Verification items for the finished model (mm, model axes). A direction names the side the tool comes from. Round coordinates to 2 decimals unless told otherwise and drop trailing zeros. Order: outer loops, then holes, each group sorted by start corner. A loop starts at its lowest first (then second) coordinate and runs counter-clockwise, first axis right, second up.
```python
from build123d import *

# Parameters (mm, degrees)
SKETCH1_W           = 45
SKETCH1_H           = 18
BOSS_EXTRUDE1_DEPTH = 3
SKETCH2_W           = 30
SKETCH2_H           = 18
BOSS_EXTRUDE3_DEPTH = 25
SKETCH5_R           = 5.5
CUT_EXTRUDE3_DEPTH  = 25
SKETCH6_R           = 11.35
CUT_EXTRUDE4_DEPTH  = 5
FILLET2_R           = 10
SKETCH7_W           = 45
SKETCH7_H           = 18
BOSS_EXTRUDE4_DEPTH = 4
SKETCH8_W           = 45
SKETCH8_H           = 18
BOSS_EXTRUDE5_DEPTH = 3.7


with BuildPart() as part:
    # Sketch1 → Boss-Extrude1 (new body)
    with BuildSketch(Plane(origin=(0, 0, 0), x_dir=(1, 0, 0), z_dir=(0, 1, 0))):
        Rectangle(SKETCH1_W, SKETCH1_H)
    extrude(amount=BOSS_EXTRUDE1_DEPTH)

    # Sketch2 → Boss-Extrude3 (add)
    with BuildSketch(Plane(origin=(0, 3, 0), x_dir=(1, 0, 0), z_dir=(0, 1, 0))):
        Rectangle(SKETCH2_W, SKETCH2_H)
    extrude(amount=BOSS_EXTRUDE3_DEPTH)

    # Sketch5 → Cut-Extrude3 (cut)
    with BuildSketch(Plane.XY.offset(9)):
        with Locations((0, 15.5)):
            Circle(SKETCH5_R)
    extrude(amount=-CUT_EXTRUDE3_DEPTH, mode=Mode.SUBTRACT)

    # Sketch6 → Cut-Extrude4 (cut)
    with BuildSketch(Plane.XY.offset(9)):
        with Locations((0, 15.5)):
            Circle(SKETCH6_R)
    extrude(amount=-CUT_EXTRUDE4_DEPTH, mode=Mode.SUBTRACT)

    # Fillet2
    fillet2_edges = [part.edges().sort_by_distance(p)[0] for p in [
        (15, 28, 0),
        (-15, 28, 0),
    ]]
    fillet(fillet2_edges, radius=FILLET2_R)

    # Sketch7 → Boss-Extrude4 (add)
    with BuildSketch(Plane.XZ):
        Rectangle(SKETCH7_W, SKETCH7_H)
    extrude(amount=BOSS_EXTRUDE4_DEPTH)

    # Sketch8 → Boss-Extrude5 (add)
    with BuildSketch(Plane.XZ.offset(4)):
        Rectangle(SKETCH8_W, SKETCH8_H)
    extrude(amount=BOSS_EXTRUDE5_DEPTH)


solid = part.part
```
1) Sectioned sample at B-B on z = 1.75. Record the cut outline in (x, y), then the cut area to 3 significant figures.
2) Sectioned sample at D-D on x = -9. Record the cut outline in (y, z).
3) Scan lines: probe 1 along Y at (x, z) = (0, 5.05); probe 2 along Y at (x, z) = (0, 1); probe 3 along Z at (x, y) = (-9, 10). Record each from-to range of solid material in increasing order.
4) Sectioned sample at C-C on y = 15.5. Record the cut outline in (x, z).
5) Draft check along Y on faces 1 (the flat face through (-15, 10, 0)), 2 (the flat face through (0, -7.7, 0)), 3 (the flat face through (2, 21, 4)), 4 (the flat face through (-19, 3, 0)). Enter one of: released by +Y, released by -Y, zero draft, split by the parting line, or undercut.
6) Go/stop test with flat-tipped pins: pin 1 Ø1.5 at (x, z) = (18, -2) entering from +Y; pin 2 Ø6 at (x, z) = (17, 1) entering from +Y; pin 3 Ø5 at (y, z) = (22, 6.5) entering from -X; pin 4 Ø12.5 at (x, y) = (0, 15.5) entering from -Z. Record where each tip stops, or that it passes through.
7) Tool access check on faces 5 (the cylindrical face through (6.1, 25.07, 6.54)), 6 (the flat face through (15, 10, 0)), 7 (the flat face through (22.5, -2, 0)). Record the directions out of +Z, -Z, +X, -X, +Y, -Y that give a thin tool (end or side, any length) a straight path to the whole face; none if there is none.
8) Sectioned sample at A-A on x = 0. Record the cut outline in (y, z).
Returned:
1. outline: (-22.5, -7.7) - (22.5, -7.7) - (22.5, 3) - (15, 3) - (15, 18) arc R10 ccw to (5, 28) - (-5, 28) arc R10 ccw to (-15, 18) - (-15, 3) - (-22.5, 3) - close; hole circle Ø11 at (0, 15.5)
1. area: 1,090 mm2
2. outline: (-7.7, -9) - (27.17, -9) - (27.17, 9) - (22.42, 9) - (22.42, 4) - (8.58, 4) - (8.58, 9) - (-7.7, 9) - close
3. probe 1: y = -7.7 to 4.15, 26.85 to 28
3. probe 2: y = -7.7 to 10, 21 to 28
3. probe 3: z = -9 to 4
4. outline: (-15, -9) - (-5.5, -9) - (-5.5, 4) - (-11.35, 4) - (-11.35, 9) - (-15, 9) - close; (5.5, -9) - (15, -9) - (15, 9) - (11.35, 9) - (11.35, 4) - (5.5, 4) - close
5. face 1: zero draft
5. face 2: released by -Y
5. face 3: undercut
5. face 4: released by +Y
6. pin 1: stops at y = 3
6. pin 2: stops at y = 22.36
6. pin 3: stops at x = -14.89
6. pin 4: stops at z = -9
7. face 5: +Z
7. face 6: +Z, -Z, +X, +Y
7. face 7: +Z, -Z, +X, +Y, -Y
8. outline: (-7.7, -9) - (10, -9) - (10, 4) - (4.15, 4) - (4.15, 9) - (-7.7, 9) - close; (21, -9) - (28, -9) - (28, 9) - (26.85, 9) - (26.85, 4) - (21, 4) - close
